```python
from build123d import *

# Parameters (mm, degrees)
SKETCH1_R           = 0.75
BOSS_EXTRUDE1_DEPTH = 0.3
FILLET1_R           = 0.3
BOSS_EXTRUDE2_DEPTH = 1
FILLET2_R           = 0.5


with BuildPart() as part:
    # Sketch1 → Boss-Extrude1 (new body)
    with BuildSketch(Plane.XY):
        with BuildLine():
            Line((-4.8, 4.4), (4.8, 4.4))
            Line((4.8, 4.4), (4.8, -4.4))
            Line((4.8, -4.4), (1.5, -4.4))
            Line((1.5, -4.4), (1.5, -8.4))
            ThreePointArc((1.5, -8.4), (0, -9.9), (-1.5, -8.4))
            Line((-1.5, -8.4), (-1.5, -4.4))
            Line((-1.5, -4.4), (-4.8, -4.4))
            Line((-4.8, -4.4), (-4.8, 4.4))
        make_face()
        with Locations((0, -8.4)):
            Circle(SKETCH1_R, mode=Mode.SUBTRACT)
    extrude(amount=BOSS_EXTRUDE1_DEPTH)

    # Fillet1
    fillet1_edges = [part.edges().sort_by_distance(p)[0] for p in [
        (-4.8, -4.4, 0.15),
        (-4.8, 4.4, 0.15),
        (4.8, 4.4, 0.15),
        (4.8, -4.4, 0.15),
        (1.5, -4.4, 0.15),
        (-1.5, -4.4, 0.15),
    ]]
    fillet(fillet1_edges, radius=FILLET1_R)

    # Sketch2 → Boss-Extrude2 (add)
    with BuildSketch(Plane(origin=(4.8, 0, 0), x_dir=(0, 0, -1), z_dir=(1, 0, 0))):
        Polygon((-0.3, -1.9), (-1.5, -0.171055671), (-1.253545223, 0), (-0.3, -1.373855504), align=None)
    boss_extrude2 = extrude(amount=-BOSS_EXTRUDE2_DEPTH)

    # Mirror1: Boss-Extrude2 across plane
    add(boss_extrude2.mirror(Plane(origin=(0, 0, 0), x_dir=(0, 0, 1), z_dir=(1, 0, 0))))

    # Sketch3 → Revolve1 (revolve)
    with BuildSketch(Plane(origin=(0, 0, 0), x_dir=(0, 0, -1), z_dir=(1, 0, 0))):
        Polygon((-1.8, 0.6), (-1.8, 1.9), (-0.3, 3.4), (-0.3, 0.6), align=None)
    revolve(axis=Axis((0, 0.6, 0.3), (0, 0, 1)))

    # Fillet2
    fillet2_edges = [part.edges().sort_by_distance(p)[0] for p in [
        (0, -0.7, 1.8),
        (0, -2.2, 0.3),
    ]]
    fillet(fillet2_edges, radius=FILLET2_R)


solid = part.part
```
The model under review builds one solid part; all positions refer to its coordinate system, in mm. A direction names the side the tool comes from. Give positions to 0.01 mm unless a question says otherwise; leave off trailing zeros. Write each loop counter-clockwise with the first axis right and the second up, starting at its lowest first coordinate (ties: lowest second). Pieces come first, ordered by that corner, then holes. Notation, with made-up numbers: (81.25, 87) - (133.25, 87) arc R3 ccw to (133.25, 91) - close; hole circle Ø3 at (10, 83.5). An arc over 180 degrees is marked (long way). Answer in a Markdown table with one row per item. Add a question column.
1. We need section B-B on y = 0.6. Write out the cut boundary in (x, z), then the cut area to 3 significant figures.
2. Insertion check: P1, Ø2, axis at x = 0, y = -8.4, coming from the -Z side; P2, Ø1, axis at x = 2, z = 1.5, coming from the -Y side. Each pin has a flat end and moves straight along its axis. Give the tip position at first contact, or say it passes through.
3. We need section A-A on x = 0. Write out the cut boundary in (y, z), then the cut area to 3 significant figures.
4. Draft analysis for pull direction X (two halves, no side actions). For faces 1 (the cylindrical face through (0.69, -8.69, 0.15)), 2 (the flat face through (4.31, -0.68, 0.78)), 3 (the cylindrical face through (0.03, -9.9, 0.15)), state which applies: +X half, -X half, draft (parallel to the pull), parting line (faces both ways), or undercut.
5. Tool access review of faces 4 (the flat face through (0, -1, 0)), 5 (the flat face through (4.31, -1.05, 0.89)), 6 (the flat face through (-4.31, -1.05, 0.89)), 7 (the flat face through (-4.31, -0.68, 0.78)): name each direction out of +Z, -Z, +X, -X, +Y, -Y from which nothing blocks a thin tool from reaching the whole face with its end or side.
6. Wall thickness on line 1 along Y through (x, z) = (0, 0.25); line 2 along X through (y, z) = (-1.5, 0.4); line 3 along Z through (x, y) = (2, -3.25): over which ranges is each line inside the solid? List them lowest first. Write a range as [from, to].
7. We need section D-D on y = -6.25. Write out the cut boundary in (x, z), then the cut area to 3 significant figures.
8. We need section C-C on x = 3.25. Write out the cut boundary in (y, z).
Ans:
| question | item | result |
|---|---|---|
| 1 | outline | (-4.8, 0) - (4.8, 0) - (4.8, 0.3) - (3.01, 0.3) arc R0.5 cw to (2.65, 0.45) - (1.45, 1.65) arc R0.5 ccw to (1.09, 1.8) - (-1.09, 1.8) arc R0.5 ccw to (-1.45, 1.65) - (-2.65, 0.45) arc R0.5 cw to (-3.01, 0.3) - (-4.8, 0.3) - close |
| 1 | area | 9.03 mm^2 |
| 2 | P1 | stops at z = 0 |
| 2 | P2 | stops at y = -0.46 |
| 3 | outline | (-9.9, 0) - (-9.15, 0) - (-9.15, 0.3) - (-9.9, 0.3) - close; (-7.65, 0) - (4.4, 0) - (4.4, 0.3) - (3.61, 0.3) arc R0.5 cw to (3.25, 0.45) - (2.05, 1.65) arc R0.5 ccw to (1.69, 1.8) - (-0.49, 1.8) arc R0.5 ccw to (-0.85, 1.65) - (-2.05, 0.45) arc R0.5 cw to (-2.41, 0.3) - (-7.65, 0.3) - close |
| 3 | area | 9.99 mm^2 |
| 4 | face 1 | undercut |
| 4 | face 2 | draft |
| 4 | face 3 | parting line |
| 5 | face 4 | -Z, +X, -X, +Y, -Y |
| 5 | face 5 | +Z, +X, -Y |
| 5 | face 6 | +Z, -X, -Y |
| 5 | face 7 | -X, +Y |
| 6 | line 1 | y = [-9.9, -9.15], [-7.65, 4.4] |
| 6 | line 2 | x = [-4.8, -3.8], [-1.71, 1.71], [3.8, 4.8] |
| 6 | line 3 | z = [0, 0.3] |
| 7 | outline | (-1.5, 0) - (1.5, 0) - (1.5, 0.3) - (-1.5, 0.3) - close |
| 7 | area | 0.900 mm^2 |
| 8 | outline | (-4.4, 0) - (4.4, 0) - (4.4, 0.3) - (-4.4, 0.3) - close |
